```python
from build123d import *

# Parameters (mm, degrees)
SKETCH1_W      = 2.7
SKETCH1_H      = 3.805531959
SKETCH1_W_2    = 1.7
SKETCH1_R      = 1.5
SKETCH1_R_2    = 2.3
EXTRUDE1_DEPTH = 2
EXTRUDE2_START = -2
SKETCH1_4_R    = 2.3
SKETCH1_4_R_2  = 1.5
EXTRUDE2_DEPTH = 1
FILLET1_R      = 1


with BuildPart() as part:
    # Sketch1 → Extrude1 (new, symmetric)
    with BuildSketch(Plane.XY):
        with BuildLine():
            Line((12.3, -4), (12.3, -3.977371993))
            ThreePointArc((12.3, -3.977371993), (12.150426084, -3.994334975), (12, -4))
            Line((12, -4), (12.3, -4))
        make_face()
        with BuildLine():
            Line((14, -4), (14, -2))
            ThreePointArc((14, -2), (13.516575089, -3.303840481), (12.3, -3.977371993))
            Line((12.3, -3.977371993), (12.3, -4))
            Line((12.3, -4), (14, -4))
        make_face()
        with Locations((10.35, -5.902765979)):
            Rectangle(SKETCH1_W, SKETCH1_H)
        Polygon((12, -4), (11.7, -4), (11.7, -7.805531959), (12.3, -7.805531959), (12.3, -4), align=None)
        with Locations((13.15, -5.902765979)):
            Rectangle(SKETCH1_W_2, SKETCH1_H)
        with BuildLine():
            ThreePointArc((12, -4), (12.150426084, -3.994334975), (12.3, -3.977371993))
            Line((12.3, -3.977371993), (12.3, 0))
            ThreePointArc((12.3, 0), (12.144761059, -0.830662386), (11.7, -1.549193338))
            Line((11.7, -1.549193338), (11.7, -4))
            Line((11.7, -4), (12, -4))
        make_face()
        with BuildLine():
            Line((12, 4), (-12, 4))
            ThreePointArc((-12, 4), (-13.414213562, 3.414213562), (-14, 2))
            Line((-14, 2), (-14, -2))
            ThreePointArc((-14, -2), (-13.414213562, -3.414213562), (-12, -4))
            Line((-12, -4), (9, -4))
            Line((9, -4), (11.7, -4))
            Line((11.7, -4), (11.7, -1.549193338))
            ThreePointArc((11.7, -1.549193338), (7.855238941, 0.830662386), (12.3, 0))
            Line((12.3, 0), (12.3, -3.977371993))
            ThreePointArc((12.3, -3.977371993), (13.516575089, -3.303840481), (14, -2))
            Line((14, -2), (14, 2))
            ThreePointArc((14, 2), (13.414213562, 3.414213562), (12, 4))
        make_face()
        with Locations((-10, 0)):
            Circle(SKETCH1_R, mode=Mode.SUBTRACT)
        with Locations((10, 0)):
            Circle(SKETCH1_R_2)
        with Locations((10, 0)):
            Circle(SKETCH1_R, mode=Mode.SUBTRACT)
    extrude(amount=EXTRUDE1_DEPTH, both=True)

    # Sketch1_4 → Extrude2 (cut)
    with BuildSketch(Plane.XY.offset(EXTRUDE2_START)):
        with BuildLine():
            Line((12.3, -4), (12.3, -3.977371993))
            ThreePointArc((12.3, -3.977371993), (12.150426084, -3.994334975), (12, -4))
            Line((12, -4), (12.3, -4))
        make_face()
        with Locations((10, 0)):
            Circle(SKETCH1_4_R)
        with Locations((10, 0)):
            Circle(SKETCH1_4_R_2, mode=Mode.SUBTRACT)
        with BuildLine():
            ThreePointArc((12, -4), (12.150426084, -3.994334975), (12.3, -3.977371993))
            Line((12.3, -3.977371993), (12.3, 0))
            ThreePointArc((12.3, 0), (12.144761059, -0.830662386), (11.7, -1.549193338))
            Line((11.7, -1.549193338), (11.7, -4))
            Line((11.7, -4), (12, -4))
        make_face()
        Polygon((12, -4), (11.7, -4), (11.7, -7.805531959), (12.3, -7.805531959), (12.3, -4), align=None)
    extrude(amount=EXTRUDE2_DEPTH, mode=Mode.SUBTRACT)

    # Fillet1
    fillet1_edges = [part.edges().sort_by_distance(p)[0] for p in [
        (9, -5.902765979, 2),
        (-13.414213562, -3.414213562, -2),
        (-14, 0, -2),
        (11.5, -7.805531959, 2),
        (-13.414213562, 3.414213562, -2),
        (0, 4, -2),
        (13.414213562, 3.414213562, -2),
        (14, -2.902765979, -2),
        (9, -5.902765979, -2),
        (-1.5, -4, -2),
        (14, -2.902765979, 2),
        (14, -7.805531959, 0),
        (9, -7.805531959, 0),
        (9, -4, 0),
        (13.414213562, 3.414213562, 2),
        (0, 4, 2),
        (-13.414213562, 3.414213562, 2),
        (-14, 0, 2),
        (-13.414213562, -3.414213562, 2),
        (-1.5, -4, 2),
    ]]
    fillet(fillet1_edges, radius=FILLET1_R)


solid = part.part
```
Source: CAD feature listing. Evaluate the final solid. Frame: model axes, mm. A direction names the side the tool comes from. Give positions to 0.01 mm unless a question says otherwise; leave off trailing zeros. Order: outer loops, then holes, each group sorted by start corner. A loop starts at its lowest first (then second) coordinate and runs counter-clockwise, first axis right, second up. Notation, with made-up numbers: (-11.5, 32.25) -> (-0.5, 32.25) arc R17 cw to (-0.5, 58.25) -> close; hole circle Ø9 at (-1.5, 52.25). An arc over 180 degrees is marked (long way). Use a Markdown table: item, result.
Q1. Access query for faces 1 (the face through (7.889, 0.913, -1.507)), 2 (the face through (12.3, -4, -1.5)), 3 (the face through (9.285, -5.89, 1.699)), 4 (the face through (-13.4, 3.43, 0.01)), 5 (the face through (-2, -4, 0)). Directions: +Z, -Z, +X, -X, +Y, -Y. A direction counts if a zero-diameter tool reaches every point of the face in a straight line with its end or side. Return the directions, or none.
A:
| item | result |
|---|---|
| face 1 | -Z |
| face 2 | -Z, -Y |
| face 3 | +Z, -X, -Y |
| face 4 | +Z, -Z, -X, +Y |
| face 5 | +Z, -Z, -X, -Y |
Q2. Section C-C (x = -11). Return the cut outline in (y, z), and give its area (3 significant figures).
A:
| item | result |
|---|---|
| outline | (-4, -1) arc R1 ccw to (-3, -2) -> (-1.12, -2) -> (-1.12, 2) -> (-3, 2) arc R1 ccw to (-4, 1) -> close; (1.12, -2) -> (3, -2) arc R1 ccw to (4, -1) -> (4, 1) arc R1 ccw to (3, 2) -> (1.12, 2) -> close |
| area | 22.2 mm^2 |
Q3. Section D-D (y = -6.25). Return the cut outline in (x, z), and give its area (3 significant figures).
A:
| item | result |
|---|---|
| outline | (9, -1) arc R1 ccw to (10, -2) -> (11.7, -2) -> (11.7, -1) -> (12.3, -1) -> (12.3, -2) -> (13, -2) arc R1 ccw to (14, -1) -> (14, 1) arc R1 ccw to (13, 2) -> (10, 2) arc R1 ccw to (9, 1) -> close |
| area | 18.5 mm^2 |
Q4. Section A-A (z = 0.05). Return the cut outline in (x, y).
A:
| item | result |
|---|---|
| outline | (-14, -2) arc R2 ccw to (-12, -4) -> (8, -4) arc R1 cw to (9, -5) -> (9, -6.81) arc R1 ccw to (10, -7.81) -> (13, -7.81) arc R1 ccw to (14, -6.81) -> (14, 2) arc R2 ccw to (12, 4) -> (-12, 4) arc R2 ccw to (-14, 2) -> close; hole circle Ø3 at (-10, 0); hole circle Ø3 at (10, 0) |
Q5. First-contact query: P1, Ø1.5, axis at x = 8.5, z = -1, coming from the -Y side; P2, Ø1.6, axis at x = -5, z = 0, coming from the -Y side; P3, Ø1.4, axis at y = -6, z = 0, coming from the -X side; P4, Ø2.5, axis at x = -10, y = 0, coming from the -Z side. Flat tips, straight axial feed; report the tip coordinate or a pass-through.
A:
| item | result |
|---|---|
| P1 | y = -7.47 |
| P2 | y = -4 |
| P3 | x = 9 |
| P4 | through |
Q6. Material intervals for line 1 (Y direction, x = 10, z = 1.05); line 2 (X direction, y = -2, z = -1.7); line 3 (Y direction, x = 10, z = -1.6), sorted ascending. Write a range as [from, to].
A:
| item | result |
|---|---|
| line 1 | [-7.8, -1.5], [1.5, 4] |
| line 2 | [-13.71, 8.86], [11.14, 11.7], [12.3, 13.71] |
| line 3 | [-7.81, -2.3], [2.3, 3.8] |
Q7. Pull-direction query (X, two-part tool) for faces 6 (the face through (13.43, 3.4, 0.01)), 7 (the face through (-1.86, -3.699, -1.715)), 8 (the face through (10.5, -1.6, -1)); classes: +X half, -X half, draft (parallel to the pull), parting line (faces both ways), or undercut.
A:
| item | result |
|---|---|
| face 6 | +X half |
| face 7 | draft |
| face 8 | undercut |
Q8. Section B-B (y = -0.25). Return the cut outline in (x, z).
A:
| item | result |
|---|---|
| outline | (-14, -1) arc R1 ccw to (-13, -2) -> (-11.48, -2) -> (-11.48, 2) -> (-13, 2) arc R1 ccw to (-14, 1) -> close; (-8.52, -2) -> (7.71, -2) -> (7.71, -1) -> (8.52, -1) -> (8.52, 2) -> (-8.52, 2) -> close; (11.48, -1) -> (12.3, -1) -> (12.3, -2) -> (13, -2) arc R1 ccw to (14, -1) -> (14, 1) arc R1 ccw to (13, 2) -> (11.48, 2) -> close |
